```python
from build123d import *

# Parameters (mm, degrees)
F1_DEPTH      = 50
F1_DEPTH_BACK = 50
F2_R          = 5
F3_DEPTH      = 25
F3_DEPTH_BACK = 25


with BuildPart() as f1:
    # F0 (on Top) → F1 (new body, two sides)
    with BuildSketch(Plane.XY) as f1_sk:
        with BuildLine():
            ThreePointArc((20, 14.5), (19.8535533906, 14.8535533906), (19.5, 15))
            Line((19.5, 15), (-19, 15))
            ThreePointArc((-19, 15), (-19.7071067812, 14.7071067812), (-20, 14))
            Line((-20, 14), (-20, -14))
            ThreePointArc((-20, -14), (-19.7071067812, -14.7071067812), (-19, -15))
            Line((-19, -15), (19.5, -15))
            ThreePointArc((19.5, -15), (19.8535533906, -14.8535533906), (20, -14.5))
            Line((20, -14.5), (20, -12.5))
            ThreePointArc((20, -12.5), (19.8535533906, -12.1464466094), (19.5, -12))
            Line((19.5, -12), (-16.5, -12))
            ThreePointArc((-16.5, -12), (-16.8535533906, -11.8535533906), (-17, -11.5))
            Line((-17, -11.5), (-17, 11.5))
            ThreePointArc((-17, 11.5), (-16.8535533906, 11.8535533906), (-16.5, 12))
            Line((-16.5, 12), (19.5, 12))
            ThreePointArc((19.5, 12), (19.8535533906, 12.1464466094), (20, 12.5))
            Line((20, 12.5), (20, 14.5))
        make_face()
    extrude(amount=F1_DEPTH)
    extrude(f1_sk.sketch, amount=-F1_DEPTH_BACK)

    # F2 (on Front) → F3 (cut, two sides)
    with BuildSketch(Plane.XZ) as f3_sk:
        Polygon((20, 50), (-20, 50), (20, 25), align=None)
        Polygon((20, -25), (-20, -50), (20, -50), align=None)
        Circle(F2_R)
    extrude(amount=-F3_DEPTH, mode=Mode.SUBTRACT)
    extrude(f3_sk.sketch, amount=F3_DEPTH_BACK, mode=Mode.SUBTRACT)


solid = f1.part
```
Input: part model. Units: mm. Frame: model coordinates. A direction names the side the tool comes from. Round coordinates to 2 decimals unless told otherwise and drop trailing zeros. Loops run counter-clockwise (first coordinate to the right, second up) from the corner with the lowest first, then second, coordinate; pieces in that order, holes last. Notation, with made-up numbers: (40.5, 23.25) - (75.5, 23.25) arc R19 ccw to (75.5, 48.25) - close; hole circle Ø6 at (45, 47). An arc over 180 degrees is marked (long way). One line per item, written item: value. Start each with the question number.
(1) Ray query, line 1 (Y direction, x = 3.5, z = 33); line 2 (X direction, y = 11, z = -32); line 3 (X direction, y = -13, z = 0). Return the intervals inside material, ascending. Write a range as [from, to].
(2) Draft query along Y for faces 3 (the flat face through (20, 13, 0)), 4 (the flat face through (6, -12, 1)), 5 (the flat face through (-9, -15, 1)), 6 (the flat face through (5.2, 12, 0.7)). Return one class per face: +Y half, -Y half, draft (parallel to the pull), parting line (faces both ways), or undercut.
(3) Section D-D, the plane x = -6.5. Return loops of the section in (y, z), plus the area to 3 significant figures.
(4) Section B-B, the plane z = 0. Return loops of the section in (x, y), plus the area to 3 significant figures.
(5) Access query for faces 1 (the flat face through (20, -14, 0)), 2 (the flat face through (-17, 0, 1)). Directions: +Z, -Z, +X, -X, +Y, -Y. A direction counts if a zero-diameter tool reaches every point of the face in a straight line with its end or side. Return the directions, or none.
(6) Contact query for flat-ended pins moving along their axis: P1, Ø11.5, axis at y = 2, z = -16, coming from the +X side; P2, Ø10, axis at x = -13.5, y = -8, coming from the +Z side; P3, Ø8, axis at x = 0, z = 0, coming from the +Y side; P4, Ø6, axis at x = 1.5, y = -11, coming from the +Z side. Output: stop coordinate, or through.
(7) Section C-C, the plane z = 15.5. Return loops of the section in (x, y), plus the area to 3 significant figures.
(8) Section A-A, the plane x = 0. Return loops of the section in (y, z).
Results below:
1. line 1: [-15, -12], [12, 15]
1. line 2: [-20, -17]
1. line 3: [-20, -5], [5, 20]
2. face 3: draft
2. face 4: undercut
2. face 5: -Y half
2. face 6: undercut
3. outline: (-15, -41.56) - (-12, -41.56) - (-12, 41.56) - (-15, 41.56) - close; (12, -41.56) - (15, -41.56) - (15, 41.56) - (12, 41.56) - close
3. area: 499 mm^2
4. outline: (-20, -14) arc R1 ccw to (-19, -15) - (-5, -15) - (-5, -12) - (-16.5, -12) arc R0.5 cw to (-17, -11.5) - (-17, 11.5) arc R0.5 cw to (-16.5, 12) - (-5, 12) - (-5, 15) - (-19, 15) arc R1 ccw to (-20, 14) - close; (5, -15) - (19.5, -15) arc R0.5 ccw to (20, -14.5) - (20, -12.5) arc R0.5 ccw to (19.5, -12) - (5, -12) - close; (5, 12) - (19.5, 12) arc R0.5 ccw to (20, 12.5) - (20, 14.5) arc R0.5 ccw to (19.5, 15) - (5, 15) - close
4. area: 251 mm^2
5. face 1: +Z, -Z, +X, +Y, -Y
5. face 2: +Z, -Z, +X
6. P1: x = -17
6. P2: z = 49.06
6. P3: through
6. P4: z = 38.33
7. outline: (-20, -14) arc R1 ccw to (-19, -15) - (19.5, -15) arc R0.5 ccw to (20, -14.5) - (20, -12.5) arc R0.5 ccw to (19.5, -12) - (-16.5, -12) arc R0.5 cw to (-17, -11.5) - (-17, 11.5) arc R0.5 cw to (-16.5, 12) - (19.5, 12) arc R0.5 ccw to (20, 12.5) - (20, 14.5) arc R0.5 ccw to (19.5, 15) - (-19, 15) arc R1 ccw to (-20, 14) - close
7. area: 311 mm^2
8. outline: (-15, -37.5) - (-12, -37.5) - (-12, -5) - (-15, -5) - close; (-15, 5) - (-12, 5) - (-12, 37.5) - (-15, 37.5) - close; (12, -37.5) - (15, -37.5) - (15, -5) - (12, -5) - close; (12, 5) - (15, 5) - (15, 37.5) - (12, 37.5) - close
